Autodesk Inventor part; units mm, degrees
ref_plane "YZ Plane" through (0, 0, 0) normal (1, 0, 0) x (0, 1, 0)
ref_plane "XZ Plane" through (0, 0, 0) normal (0, 1, 0) x (-1, 0, 0)
ref_plane "XY Plane" through (0, 0, 0) normal (0, 0, 1) x (1, 0, 0)
sketch "Sketch1" plane through (0, 0, 0) normal (0, 0, 1) x (1, 0, 0)
  line L0 (148.5, -9.5) -> (148.5, -6.2) construction
  line L1 (148.5, -6.2) -> (193, -6.2) construction
  line L2 (193, 9.5) -> (193, -6.2) construction
  line L3 (0, 9.5) -> (193, 9.5) construction
  line L4 (0, -9.5) -> (0, 9.5) construction
  line L5 (148.5, -9.5) -> (0, -9.5) construction
  line L6 (0, 9.5) -> (193, 9.5)
  line L7 (193, 9.5) -> (193, -57.5)
  line L8 (193, -57.5) -> (0, -57.5)
  line L9 (0, -57.5) -> (0, 9.5)
  circle A0 centre (128.6667, -4.8333) radius 1.621
  circle A1 centre (96.5, 3.1667) radius 1.621
  circle A2 centre (64.3333, -4.8333) radius 1.621
  circle A3 centre (32.1667, 3.1667) radius 1.621
  circle A4 centre (32.1667, -4.8333) radius 1.621
  circle A5 centre (64.3333, 3.1667) radius 1.621
  circle A6 centre (96.5, -4.8333) radius 1.621
  circle A7 centre (128.6667, 3.1667) radius 1.621
  circle A8 centre (160.8333, 3.1667) radius 1.621
  point P0 (0, 0)
extrude "Extrusion1" add sketch "Sketch1" along normal blind 10 contours L6 L7 L8 L9 | A0 | A1 | A2 | A3 | A4 | A5 | A6 | A7 | A8
sketch "Sketch2" plane through (0, -57.5, 0) normal (-1, 0, 0) x (0, 0, 1)
  line L0 (-111.7541, 55) -> (-111.7541, 67) construction
  line L1 (-116, 67) -> (-111.7541, 67) construction
  line L2 (-116, 48) -> (-116, 67) construction
  line L3 (4, 48) -> (-116, 48) construction
  line L4 (4, 48) -> (4, 67) construction
  line L5 (-54.7541, 67) -> (4, 67) construction
  line L6 (-54.7541, 67) -> (-54.7541, 55) construction
  line L7 (-54.7541, 55) -> (-111.7541, 55) construction
  line L8 (0, 67) -> (0, 0)
  line L9 (4, 67) -> (0, 67)
  line L10 (0, 67) -> (0, 48)
  line L11 (0, 48) -> (4, 48)
  line L12 (4, 48) -> (4, 67)
  point P0 (0, 57.5)
extrude "Extrusion2" cut sketch "Sketch2" against normal through all
sketch "Sketch3" plane through (0, 0, 10) normal (0, 0, 1) x (1, 0, 0)
  line L0 (193, -9.5) -> (193, 9.5)
  line L1 (0, -9.5) -> (193, -9.5)
  line L2 (0, 9.5) -> (0, -9.5)
  line L3 (193, 9.5) -> (0, 9.5)
  line L4 (0, 0) -> (193, 0) construction
  point P0 (32.1667, 3.1667)
  point P1 (64.3333, 3.1667)
  point P2 (96.5, 3.1667)
  point P3 (128.6667, 3.1667)
  point P4 (160.8333, 3.1667)
  point P5 (32.1667, -4.8333)
  point P6 (64.3333, -4.8333)
  point P7 (96.5, -4.8333)
  point P8 (128.6667, -4.8333)
  point P9 (160.8333, -4.8333)
  dimension "d4" = 32.1667
  dimension "d5" = 32.1667
  dimension "d6" = 32.1667
  dimension "d7" = 32.1667
  dimension "d8" = 32.1667
  dimension "d9" = 8
  dimension "d10" = 6.3333
hole "Hole1" at (32.1667, 3.1667, 10) at (64.3333, 3.1667, 10) at (96.5, 3.1667, 10) at (128.6667, 3.1667, 10) at (160.8333, 3.1667, 10) at (32.1667, -4.8333, 10) at (64.3333, -4.8333, 10) at (96.5, -4.8333, 10) at (128.6667, -4.8333, 10) direction (0, 0, -1) diameter 4.5 depth 14.2 counterbore diameter 8 counterbore depth 4.6
properties part number "foot bracket foot backside"
Input: part model. Units: mm. Frame: model coordinates. A direction names the side the tool comes from. Coordinates: 2 decimals unless noted, no trailing zeros. Loops run counter-clockwise (first coordinate to the right, second up) from the corner with the lowest first, then second, coordinate; pieces in that order, holes last.
Q1. Material intervals for line 1 (X direction, y = 4, z = 8.25); line 2 (Y direction, x = 111, z = 2.5), sorted ascending.
Q2. Set-up query: faces 4 (the face through (157.46, 1.02, 7.67)), 5 (the face through (34.363, -4.346, 4.69)), 6 (the face through (95, -9.5, 2)). Return all of +Z, -Z, +X, -X, +Y, -Y with unobstructed straight access to the full face (end or side cutting, diameter ignored); none if empty.
Q3. Cut plane A-A (x = 52.5). Output: boundary loops of the cut face in (y, z).
Q4. Contact query for flat-ended pins moving along their axis: pin 1 (4 mm diameter, centred on x = 59, z = 1.5, fed in from +Y); pin 2 (6 mm diameter, centred on x = 96.5, y = -4.83, fed in from -Z); pin 3 (7 mm diameter, centred on x = 64.33, y = -4.83, fed in from +Z). Output: stop coordinate, or through.
Q5. Draft query along Y for faces 1 (the face through (95, 9.5, 7)), 2 (the face through (62.102, -4.54, 4.69)), 3 (the face through (95, -33, 0)). Return one class per face: +Y half, -Y half, draft (parallel to the pull), parting line (faces both ways), or undercut.
Working result:
1. line 1: x = 0 to 28.25, 36.08 to 60.42, 68.25 to 92.59, 100.41 to 124.75, 132.58 to 156.92, 164.75 to 193
1. line 2: y = -57.5 to -9.5
2. face 4: +Z
2. face 5: +Z, -Z
2. face 6: -Z, +X, -X, +Y
3. outline: (-57.5, 0) - (-9.5, 0) - (-9.5, 4) - (9.5, 4) - (9.5, 10) - (-57.5, 10) - close
4. pin 1: stops at y = -9.5
4. pin 2: stops at z = 4
4. pin 3: stops at z = 5.4
5. face 1: +Y half
5. face 2: undercut
5. face 3: draft
